Design review of the part built by this model. Coordinates are the model's own, in mm. Face numbers are marked on the shaded views. A direction names the side the tool comes from. Give positions to 0.01 mm unless a question says otherwise; leave off trailing zeros. Write each loop counter-clockwise with the first axis right and the second up, starting at its lowest first coordinate (ties: lowest second). Pieces come first, ordered by that corner, then holes. Notation, with made-up numbers: (73.5, 35.25) - (103.5, 35.25) arc R16 ccw to (103.5, 62.25) - close; hole circle Ø4 at (-24, 88.5). An arc over 180 degrees is marked (long way). Use a Markdown table: item, result. Add a question column.
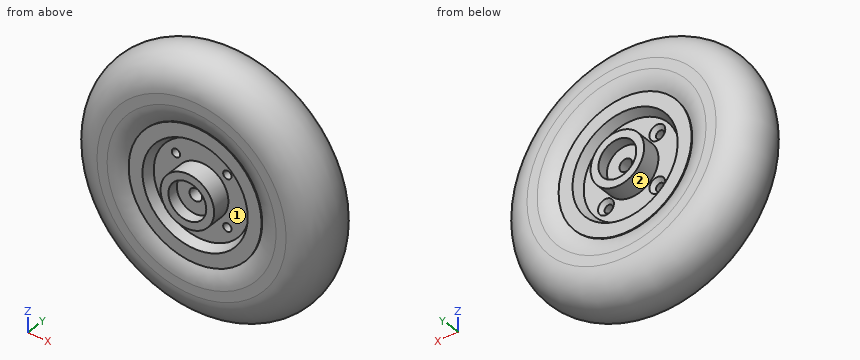
```python
from build123d import *

# Parameters (mm, degrees)
HOLE_WIZARD_M6_1_D           = 6.6
HOLE_WIZARD_M6_1_CSINK_D     = 12.6
HOLE_WIZARD_M6_1_CSINK_ANGLE = 90


with BuildPart() as part:
    # 草圖1 → 旋轉1 (revolve)
    with BuildSketch(Plane.XY):
        Polygon((15, 29.5), (21.25, 29.5), (21.25, 14.25), (38, 14.25), (41.75, 21.25), (52.75, 21.25), (52.75, -21.25), (41.75, -21.25), (38, -14.25), (21.25, -14.25), (21.25, -29.5), (15, -29.5), (15, -20.5), (5, -20.5), (5, 20.5), (15, 20.5), align=None)
    revolve(axis=Axis((0, 152.231132075, 0), (0, -1, 0)))

    # 草圖2 → 旋轉2 (revolve)
    with BuildSketch(Plane.XY):
        with BuildLine():
            Line((-75, 25), (-67, 25))
            ThreePointArc((-67, 25), (-42, 0), (-67, -25))
            Line((-67, -25), (-75, -25))
            ThreePointArc((-75, -25), (-100, 0), (-75, 25))
        make_face()
    revolve(axis=Axis((0, 0, 0), (0, 1, 0)))

    # M6 平錐坑頭螺釘的錐孔1 (through all)
    with Locations(Plane(origin=(0, 14.25, 0), x_dir=(1, 0, 0), z_dir=(0, 1, 0))):
        with Locations((-20.375, -20.375), (-20.375, 20.375), (20.375, -20.375), (20.375, 20.375)):
            CounterSinkHole(HOLE_WIZARD_M6_1_D / 2, HOLE_WIZARD_M6_1_CSINK_D / 2, counter_sink_angle=HOLE_WIZARD_M6_1_CSINK_ANGLE)


solid = part.part
```
(1) For line 1 along X through (y, z) = (-22, 4); line 2 along X through (y, z) = (13.5, 17); line 3 along Z through (x, y) = (0, -26), list the stretches that pass through material, from the lowest coordinate up.
(2) Insertion check: pin 1 (10.5 mm diameter, centred on x = -20.375, z = 20.375, fed in from -Y); pin 2 (5 mm diameter, centred on x = 7, y = -19, fed in from -Z); pin 3 (23 mm diameter, centred on x = 0, z = 5.5, fed in from -Y); pin 4 (1 mm diameter, centred on x = 49.5, y = -9.5, fed in from +Z). Each pin has a flat end and moves straight along its axis. Give the tip position at first contact, or say it passes through.
(3) Add section B-B (y = -17). State the section outline as (x, z) points, and give its area (3 significant figures).
(4) Add section A-A (y = 5.5). State the section outline as (x, z) points (1 decimal), and give its area (3 significant figures).
(5) Tool access review of the marked faces 1 and 2: name each direction out of +Z, -Z, +X, -X, +Y, -Y from which nothing blocks a thin tool from reaching the whole face with its end or side.
Answers follow:
| question | item | result |
|---|---|---|
| 1 | line 1 | -86.78 to -54.98, -20.87 to -14.46, 14.46 to 20.87, 54.98 to 86.78 |
| 1 | line 2 | -94.53 to -24.78, -15.97 to 15.97, 24.78 to 94.53 |
| 1 | line 3 | -21.25 to -15, 15 to 21.25 |
| 2 | pin 1 | y = -14.25 |
| 2 | pin 2 | z = -93.53 |
| 2 | pin 3 | y = -29.5 |
| 2 | pin 4 | z = 85.1 |
| 3 | outline | circle Ø186.66 at (0, 0); circle Ø42.5 at (0, 0); hole circle Ø78.95 at (0, 0); hole circle Ø10 at (0, 0) |
| 3 | area | 23,800 mm^2 |
| 4 | outline | circle Ø198.8 at (0, 0); hole circle Ø6.6 at (-20.4, -20.4); hole circle Ø6.6 at (-20.4, 20.4); hole circle Ø10 at (0, 0); hole circle Ø6.6 at (20.4, -20.4); hole circle Ø6.6 at (20.4, 20.4) |
| 4 | area | 30,800 mm^2 |
| 5 | face 1 | -Y |
| 5 | face 2 | +Y |
